from build123d import *

# Parameters (mm, degrees)
SKETCH2_W           = 50
SKETCH2_H           = 50
SKETCH2_R           = 1.5
SKETCH2_R_2         = 1.25
BOSS_EXTRUDE1_DEPTH = 3
SKETCH3_W           = 10
SKETCH3_H           = 10
SKETCH3_R           = 1.5
BOSS_EXTRUDE2_DEPTH = 30
FILLET2_R           = 5
FILLET3_R           = 5


with BuildPart() as part:
    # Sketch2 → Boss-Extrude1 (new body)
    with BuildSketch(Plane.XY):
        with Locations((-41.57818593, 67.684487612)):
            Rectangle(SKETCH2_W, SKETCH2_H)
        with Locations((-61.57818593, 87.684487612)):
            Circle(SKETCH2_R, mode=Mode.SUBTRACT)
        with Locations((-21.57818593, 87.684487612)):
            Circle(SKETCH2_R, mode=Mode.SUBTRACT)
        with Locations((-61.57818593, 47.684487612)):
            Circle(SKETCH2_R, mode=Mode.SUBTRACT)
        with Locations((-21.57818593, 47.684487612)):
            Circle(SKETCH2_R, mode=Mode.SUBTRACT)
        with Locations((-41.57818593, 67.684487612)):
            Circle(SKETCH2_R_2, mode=Mode.SUBTRACT)
    extrude(amount=BOSS_EXTRUDE1_DEPTH)

    # Sketch3 → Boss-Extrude2 (add)
    # profile 1 of 4: a face of its own
    with BuildSketch(Plane.XY.offset(3)):
        with Locations((-61.57818593, 87.684487612)):
            Rectangle(SKETCH3_W, SKETCH3_H)
        with Locations((-61.57818593, 87.684487612)):
            Circle(SKETCH3_R, mode=Mode.SUBTRACT)
    # profile 2 of 4: a face of its own
    with BuildSketch(Plane.XY.offset(3)):
        with Locations((-21.57818593, 87.684487612)):
            Rectangle(SKETCH3_W, SKETCH3_H)
        with Locations((-21.57818593, 87.684487612)):
            Circle(SKETCH3_R, mode=Mode.SUBTRACT)
    # profile 3 of 4: a face of its own
    with BuildSketch(Plane.XY.offset(3)):
        with Locations((-21.57818593, 47.684487612)):
            Rectangle(SKETCH3_W, SKETCH3_H)
        with Locations((-21.57818593, 47.684487612)):
            Circle(SKETCH3_R, mode=Mode.SUBTRACT)
    # profile 4 of 4: a face of its own
    with BuildSketch(Plane.XY.offset(3)):
        with Locations((-61.57818593, 47.684487612)):
            Rectangle(SKETCH3_W, SKETCH3_H)
        with Locations((-61.57818593, 47.684487612)):
            Circle(SKETCH3_R, mode=Mode.SUBTRACT)
    extrude(amount=BOSS_EXTRUDE2_DEPTH)

    # Fillet2
    fillet2_edges = [part.edges().sort_by_distance(p)[0] for p in [
        (-16.57818593, 42.684487612, 16.5),
        (-66.57818593, 42.684487612, 16.5),
        (-66.57818593, 92.684487612, 16.5),
        (-16.57818593, 92.684487612, 16.5),
    ]]
    fillet(fillet2_edges, radius=FILLET2_R)

    # Fillet3
    fillet3_edges = [part.edges().sort_by_distance(p)[0] for p in [
        (-16.57818593, 82.684487612, 18),
        (-26.57818593, 82.684487612, 18),
        (-26.57818593, 92.684487612, 18),
        (-16.57818593, 52.684487612, 18),
        (-26.57818593, 52.684487612, 18),
        (-26.57818593, 42.684487612, 18),
        (-56.57818593, 42.684487612, 18),
        (-56.57818593, 52.684487612, 18),
        (-66.57818593, 52.684487612, 18),
        (-66.57818593, 82.684487612, 18),
        (-56.57818593, 82.684487612, 18),
        (-56.57818593, 92.684487612, 18),
    ]]
    fillet(fillet3_edges, radius=FILLET3_R - 0.0001)  # a hair under: the kernel refuses the full size


solid = part.part
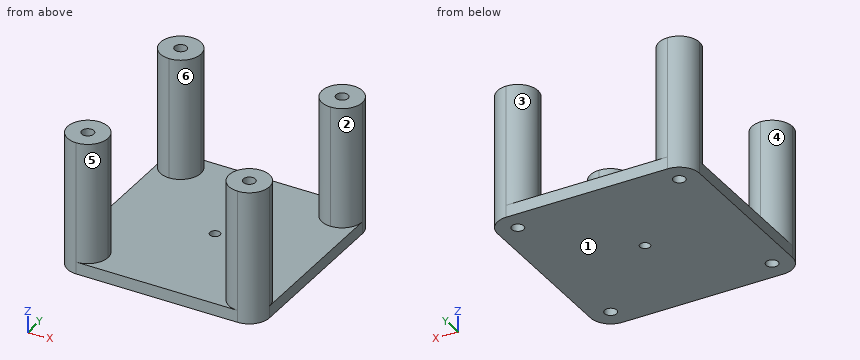
Geometry: final body of the model. Coordinates: model frame, mm. Face numbers are marked on the shaded views. A direction names the side the tool comes from. Give positions to 0.01 mm unless a question says otherwise; leave off trailing zeros. Loops run counter-clockwise (first coordinate to the right, second up) from the corner with the lowest first, then second, coordinate; pieces in that order, holes last. Notation, with made-up numbers: (-13.5, 45) - (0.5, 45) arc R24 ccw to (0.5, 76) - close; hole circle Ø3 at (-33.75, 5.25). An arc over 180 degrees is marked (long way). Answer as CSV lines item,"result". Start each with the question number.
1. Pin query (flat end, axial travel): P1, Ø1.8, axis at x = -21.58, y = 87.68, coming from the -Z side; P2, Ø10, axis at x = -57, y = 74, coming from the +Z side; P3, Ø3, axis at x = -24.5, z = 21, coming from the +Y side. Return the tip coordinate at first contact, or that it passes through.
2. Ray query, L1, parallel to X at y = 88.5, z = 15.5; L2, parallel to X at y = 86.5, z = 8.5; L3, parallel to Z at x = -43, y = 45. Return the intervals inside material, ascending.
3. Reachability of the marked faces 4, 5 and 6 from +Z, -Z, +X, -X, +Y, -Y: full face, straight path, thin tool, end or side. Return the list, or none.
4. Section C-C, the plane y = 54.5. Return loops of the section in (x, z).
5. Section D-D, the plane x = -51.5. Return loops of the section in (y, z), plus the area to 3 significant figures.
6. Section B-B, the plane x = -24. Return loops of the section in (y, z), plus the area to 3 significant figures.
7. Draft query along Y for the marked faces 1, 2 and 3. Return one class per face: released by +Y, released by -Y, zero draft, split by the parting line, or undercut.
8. Section A-A, the plane z = 4. Give the number of separate pieces and of enclosed holes in the cut face, plus the area to 3 significant figures.
Answers:
1,P1,"passes through"
1,P2,"stops at z = 3"
1,P3,"stops at y = 92.48"
2,L1,"x = -66.51 to -62.84, -60.32 to -56.65, -26.51 to -22.84, -20.32 to -16.65"
2,L2,"x = -66.44 to -62.5, -60.66 to -56.72, -26.44 to -22.5, -20.66 to -16.72"
2,L3,"z = 0 to 3"
3,face 4,"+Z, -X"
3,face 5,"+Z, -Y"
3,face 6,"+Z"
4,outline,"(-66.58, 0) - (-16.58, 0) - (-16.58, 3) - (-66.58, 3) - close"
5,outline,"(42.68, 0) - (92.68, 0) - (92.68, 3) - (42.68, 3) - close"
5,area,"150 mm2"
6,outline,"(42.68, 0) - (92.68, 0) - (92.68, 3) - (92.06, 3) - (92.06, 33) - (83.31, 33) - (83.31, 3) - (52.06, 3) - (52.06, 33) - (43.31, 33) - (43.31, 3) - (42.68, 3) - close"
6,area,"675 mm2"
7,face 1,"zero draft"
7,face 2,"undercut"
7,face 3,"released by +Y"
8,separate pieces,"4"
8,enclosed holes,"4"
8,area,"286 mm2"
